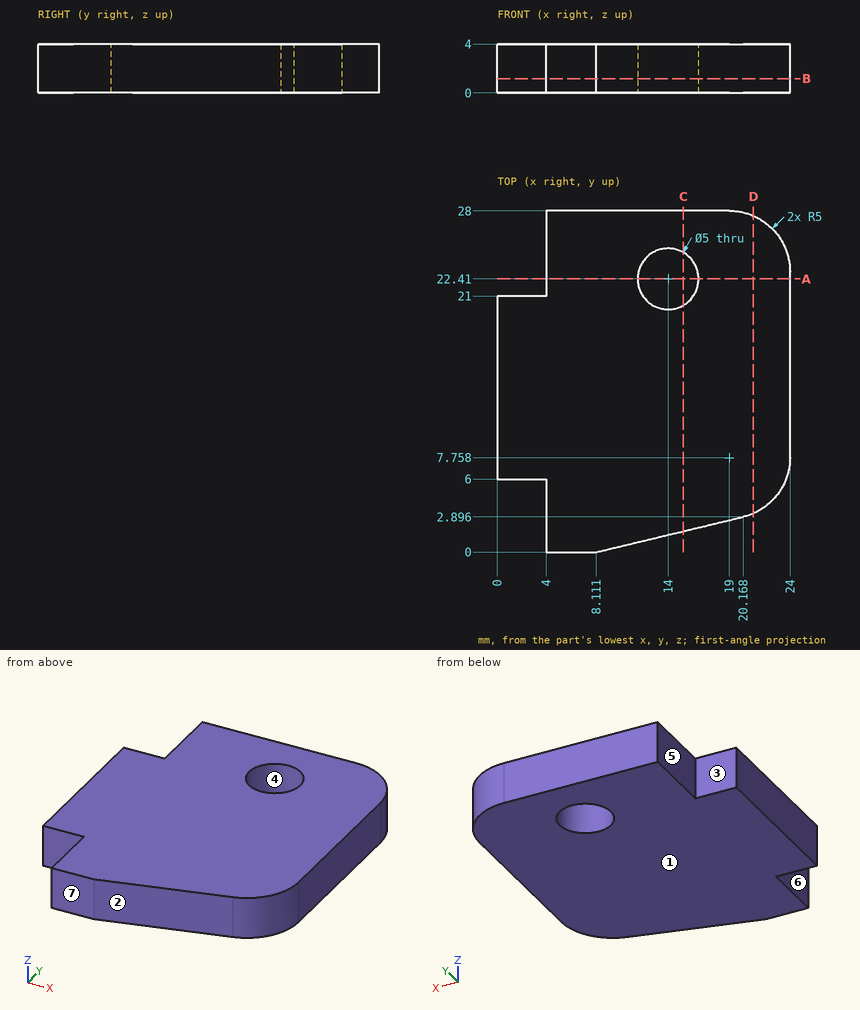
Here's the drawing with two shaded views (mm, measured from the low corner). I have some questions. A direction names the side the tool comes from. Round coordinates to 2 decimals unless told otherwise and drop trailing zeros. Loops run counter-clockwise (first coordinate to the right, second up) from the corner with the lowest first, then second, coordinate; pieces in that order, holes last. Notation, with made-up numbers: (11, 74) - (56, 74) arc R22 ccw to (56, 93) - close; hole circle Ø2 at (15.5, -5). An arc over 180 degrees is marked (long way). Use CSV: the item, a comma, the result in double quotes. Start each with the question number.
1) Please list where these lines run through material, in increasing order: probe 1 along Y at (x, z) = (14, 2.5) (1 decimal); probe 2 along Y at (x, z) = (3.75, 0.5); probe 3 along X at (y, z) = (4.75, 1.7) (1 decimal). Write a range as [from, to].
2) We'd pull the mould along Y, two halves only. Please class the marked faces 1, 2, 3 and 4: released by +Y, released by -Y, zero draft, split by the parting line, or undercut.
3) For pin 1 Ø4 at (x, y) = (14, 22.41) entering from -Z; pin 2 Ø1.2 at (x, z) = (1, 1.5) entering from -Y, each with a flat end and sliding along its axis, tell me the tip position at first contact or that it passes through.
4) If we section it at B-B on z = 1.15: Write out the boundary of the cut face in (x, y).
5) For the marked faces 5, 6 and 7, which set-ups out of +Z, -Z, +X, -X, +Y, -Y let a thin tool reach every point of the face, with its end or its side?
6) If we section it at C-C on x = 15.25: Write out the boundary of the cut face in (y, z) (1 decimal), plus the area to 3 significant figures.
7) If we section it at A-A on y = 22.41: Write out the boundary of the cut face in (x, z), plus the area to 3 significant figures.
8) If we section it at D-D on x = 21: Write out the boundary of the cut face in (y, z) (1 decimal).
Geometry results:
1,probe 1,"y = [1.4, 19.9], [24.9, 28]"
1,probe 2,"y = [6, 21]"
1,probe 3,"x = [4, 23]"
2,face 1,"zero draft"
2,face 2,"released by -Y"
2,face 3,"released by +Y"
2,face 4,"undercut"
3,pin 1,"passes through"
3,pin 2,"stops at y = 6"
4,outline,"(0, 6) - (4, 6) - (4, 0) - (8.11, 0) - (20.17, 2.9) arc R5 ccw to (24, 7.76) - (24, 23) arc R5 ccw to (19, 28) - (4, 28) - (4, 21) - (0, 21) - close; hole circle Ø5 at (14, 22.41)"
5,face 5,"+Z, -Z, -X, +Y"
5,face 6,"+Z, -Z, -X, -Y"
5,face 7,"+Z, -Z, +X, -X, -Y"
6,outline,"(1.7, 0) - (20.2, 0) - (20.2, 4) - (1.7, 4) - close; (24.6, 0) - (28, 0) - (28, 4) - (24.6, 4) - close"
6,area,"87.8 mm2"
7,outline,"(4, 0) - (11.5, 0) - (11.5, 4) - (4, 4) - close; (16.5, 0) - (24, 0) - (24, 4) - (16.5, 4) - close"
7,area,"60.0 mm2"
8,outline,"(3.2, 0) - (27.6, 0) - (27.6, 4) - (3.2, 4) - close"
